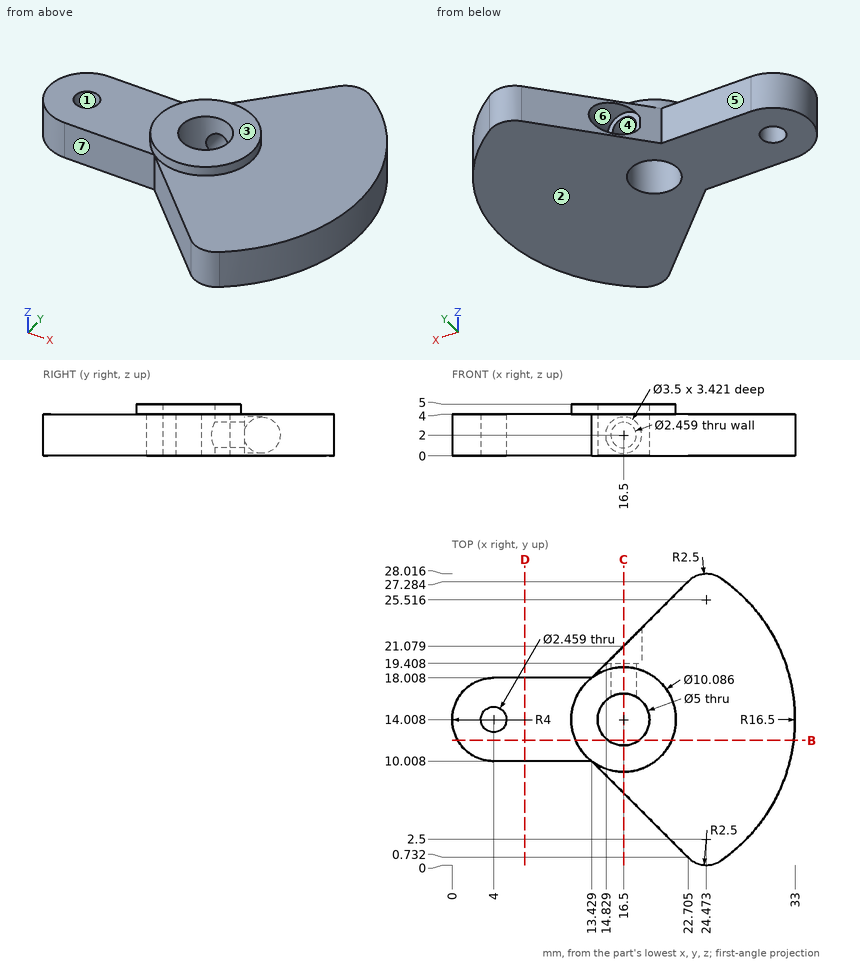
Geometry: see drawing. Coordinates: mm, zero at the bounding-box minimum. A direction names the side the tool comes from. Round coordinates to 2 decimals unless told otherwise and drop trailing zeros. Write each loop counter-clockwise with the first axis right and the second up, starting at its lowest first coordinate (ties: lowest second). Pieces come first, ordered by that corner, then holes.
Item 1: Section query B-B (y = 12). Return loops of the section in (x, z), plus the area to 3 significant figures.
Item 2: Material intervals for L1, parallel to Z at x = 16.5, y = 17.95; L2, parallel to Y at x = 4, z = 0.9; L3, parallel to Z at x = 23, y = 10.25, sorted ascending.
Item 3: Mould query, pull axis Z, two halves, no side actions, for the marked faces 1, 2, 3 and 4. Classes: +Z half, -Z half, draft (parallel to the pull), parting line (faces both ways), or undercut.
Item 4: Section query C-C (x = 16.5). Give the number of separate pieces and of enclosed holes in the cut face.
Item 5: Pin query (flat end, axial travel): P1, Ø4, axis at x = 6.5, y = 14.5, coming from the +Z side; P2, Ø2, axis at x = 16.5, z = 2, coming from the +Y side; P3, Ø1.2, axis at x = 11, z = 2.5, coming from the -Y side; P4, Ø4.5, axis at x = 16.5, y = 14.01, coming from the +Z side. Return the tip coordinate at first contact, or that it passes through.
Item 6: Section query D-D (x = 7). Return loops of the section in (y, z).
Item 7: Set-up query: the marked faces 5, 6 and 7. Return all of +Z, -Z, +X, -X, +Y, -Y with unobstructed straight access to the full face (end or side cutting, diameter ignored); none if empty.
Completed:
1. outline: (0.54, 0) - (15.01, 0) - (15.01, 5) - (11.87, 5) - (11.87, 4) - (0.54, 4) - close; (17.99, 0) - (32.88, 0) - (32.88, 4) - (21.13, 4) - (21.13, 5) - (17.99, 5) - close
1. area: 124 mm2
2. L1: z = 0 to 0.77, 3.23 to 5
2. L2: y = 10.01 to 12.78, 15.24 to 18.01
2. L3: z = 0 to 4
3. face 1: draft
3. face 2: -Z half
3. face 3: +Z half
3. face 4: undercut
4. separate pieces: 3
4. enclosed holes: 0
5. P1: stops at z = 4
5. P2: stops at y = 11.72
5. P3: stops at y = 10.01
5. P4: passes through
6. outline: (10.01, 0) - (18.01, 0) - (18.01, 4) - (10.01, 4) - close
7. face 5: +Z, -Z, -X, +Y
7. face 6: +Y
7. face 7: +Z, -Z, -X, -Y
